```python
from build123d import *

# Parameters (mm, degrees)
SKETCH_1_W           = 100
SKETCH_1_H           = 30
SKETCH_1_R           = 1.45
EXTRUDE_1_DEPTH      = 10
SKETCH_2_W           = 24
SKETCH_2_H           = 30
CUT_EXTRUDE_1_DEPTH  = 6.5
SKETCH_3_W           = 9
SKETCH_3_H           = 15
CUT_EXTRUDE_2_DEPTH  = 16.5
SKETCH_4_W           = 9
SKETCH_4_H           = 4
CUT_EXTRUDE_3_DEPTH  = 16.5
SKETCH_6_R           = 1.5
CUT_EXTRUDE_4_DEPTH  = 16
CUT_EXTRUDE_START    = -8
SKETCH_7_R           = 1.5
CUT_EXTRUDE_5_DEPTH  = 8
CHAMFER_1_SIZE       = 5
CUT_EXTRUDE_START_2  = -30
SKETCH_10_R          = 1.5
CUT_EXTRUDE_8_DEPTH  = 30
SKETCH_11_R          = 1.5
CUT_EXTRUDE_9_DEPTH  = 30
SKETCH_15_W          = 27.5
SKETCH_15_H          = 2.5
CUT_EXTRUDE_14_DEPTH = 30
CUT_EXTRUDE_15_REACH = 106.881
SKETCH_16_W          = 9
SKETCH_16_H          = 2
SKETCH_19_R          = 1.45
CUT_EXTRUDE_18_DEPTH = 105.880884817
SKETCH_21_W          = 30
SKETCH_21_H          = 6.5
EXTRUDE_2_DEPTH      = 3
CUT_EXTRUDE_START_3  = -2
SKETCH_22_R          = 1.5
CUT_EXTRUDE_19_DEPTH = 2
SKETCH_23_W          = 30
SKETCH_23_H          = 6.5
EXTRUDE_3_DEPTH      = 3
SKETCH_24_R          = 1.5
CUT_EXTRUDE_20_DEPTH = 2


with BuildPart() as part:
    # 草图1 → 凸台-拉伸1 (new body)
    with BuildSketch(Plane(origin=(0, 0, 0), x_dir=(1, 0, 0), z_dir=(0, 1, 0))):
        with Locations((-50, 15)):
            Rectangle(SKETCH_1_W, SKETCH_1_H)
        with Locations(Location((-50, 25, 0), (0, 0, 270))):
            Circle(SKETCH_1_R, mode=Mode.SUBTRACT)
        with Locations(Location((-50, 5, 0), (0, 0, 270))):
            Circle(SKETCH_1_R, mode=Mode.SUBTRACT)
    extrude(amount=EXTRUDE_1_DEPTH)

    # 草图2 → 切除-拉伸1 (cut)
    with BuildSketch(Plane(origin=(0, 10, 0), x_dir=(1, 0, 0), z_dir=(0, 1, 0))):
        with Locations((-50, 15)):
            Rectangle(SKETCH_2_W, SKETCH_2_H)
    extrude(amount=-CUT_EXTRUDE_1_DEPTH, mode=Mode.SUBTRACT)

    # 草图3 → 切除-拉伸2 (cut)
    with BuildSketch(Plane(origin=(0, 10, 0), x_dir=(1, 0, 0), z_dir=(0, 1, 0))):
        with Locations((-68, 22.5)):
            Rectangle(SKETCH_3_W, SKETCH_3_H)
        with Locations((-32, 22.5)):
            Rectangle(SKETCH_3_W, SKETCH_3_H)
    extrude(amount=-CUT_EXTRUDE_2_DEPTH, mode=Mode.SUBTRACT)

    # 草图4 → 切除-拉伸3 (cut)
    with BuildSketch(Plane(origin=(0, 0, -15), x_dir=(-1, 0, 0), z_dir=(0, 0, -1))):
        with Locations((68, 8)):
            Rectangle(SKETCH_4_W, SKETCH_4_H)
        with Locations((32, 8)):
            Rectangle(SKETCH_4_W, SKETCH_4_H)
    extrude(amount=-CUT_EXTRUDE_3_DEPTH, mode=Mode.SUBTRACT)

    # 草图6 → 切除-拉伸4 (cut)
    with BuildSketch(Plane(origin=(-62, 0, 0), x_dir=(0, 0, -1), z_dir=(1, 0, 0))):
        with Locations((22.5, 5)):
            Circle(SKETCH_6_R)
    extrude(amount=-CUT_EXTRUDE_4_DEPTH, mode=Mode.SUBTRACT)

    # 草图7 → 切除-拉伸5 (cut)
    with BuildSketch(Plane.ZY.offset(38).offset(CUT_EXTRUDE_START)):
        with Locations(Location((-22.5, 5, 0), (0, 0, 180))):
            Circle(SKETCH_7_R)
    extrude(amount=CUT_EXTRUDE_5_DEPTH, mode=Mode.SUBTRACT)

    # 倒角1
    chamfer_1_edges = [part.edges().sort_by_distance(p)[0] for p in [
        (-32, 6, -15),
        (-68, 6, -15),
    ]]
    chamfer(chamfer_1_edges, length=CHAMFER_1_SIZE)

    # 草图10 → 切除-拉伸8 (cut)
    with BuildSketch(Plane(origin=(-100, -149.284504662, 244.723777946), x_dir=(0, 0, 1), z_dir=(-1, 0, 0)).offset(CUT_EXTRUDE_START_2)):
        with Locations(Location((-267.223777946, 154.284504662, 0), (0, 0, 180))):
            Circle(SKETCH_10_R)
    extrude(amount=CUT_EXTRUDE_8_DEPTH, mode=Mode.SUBTRACT)

    # 草图11 → 切除-拉伸9 (cut)
    with BuildSketch(Plane(origin=(0, -149.284504662, 244.723777946), x_dir=(0, 0, -1), z_dir=(1, 0, 0))):
        with Locations((267.223777946, 154.284504662)):
            Circle(SKETCH_11_R)
    extrude(amount=-CUT_EXTRUDE_9_DEPTH, mode=Mode.SUBTRACT)

    # 草图15 → 切除-拉伸14 (cut)
    with BuildSketch(Plane(origin=(0, 0, -30), x_dir=(-1, 0, 0), z_dir=(0, 0, -1))):
        with Locations((13.75, 8.75)):
            Rectangle(SKETCH_15_W, SKETCH_15_H)
        with Locations((86.25, 8.75)):
            Rectangle(SKETCH_15_W, SKETCH_15_H)
    extrude(amount=-CUT_EXTRUDE_14_DEPTH, mode=Mode.SUBTRACT)

    # 切除-拉伸15: up to this plane
    cut_extrude_15_end = Plane(origin=(-63.5, 6, -10), z_dir=(0, -0.7071067811865456, 0.7071067811865495))
    # 草图16 → 切除-拉伸15 (cut, up to the surface)
    with BuildSketch(Plane.XY, mode=Mode.PRIVATE) as cut_extrude_15_sk1:
        with Locations((-68, 1)):
            Rectangle(SKETCH_16_W, SKETCH_16_H)
    cut_extrude_15_tool1 = split(extrude(cut_extrude_15_sk1.sketch, amount=-CUT_EXTRUDE_15_REACH, mode=Mode.PRIVATE), bisect_by=cut_extrude_15_end, keep=Keep.BOTH, mode=Mode.PRIVATE)
    add(cut_extrude_15_tool1.solids().sort_by_distance((-68, 1, 0))[0], mode=Mode.SUBTRACT)
    # 草图16 → 切除-拉伸15 (cut, up to the surface)
    with BuildSketch(Plane.XY, mode=Mode.PRIVATE) as cut_extrude_15_sk2:
        with Locations((-32, 1)):
            Rectangle(SKETCH_16_W, SKETCH_16_H)
    cut_extrude_15_tool2 = split(extrude(cut_extrude_15_sk2.sketch, amount=-CUT_EXTRUDE_15_REACH, mode=Mode.PRIVATE), bisect_by=cut_extrude_15_end, keep=Keep.BOTH, mode=Mode.PRIVATE)
    add(cut_extrude_15_tool2.solids().sort_by_distance((-32, 1, 0))[0], mode=Mode.SUBTRACT)

    # 草图19 → 切除-拉伸18 (cut, through all)
    with BuildSketch(Plane.XZ):
        with Locations(Location((-3, -3, 0), (0, 0, 270))):
            Circle(SKETCH_19_R)
        with Locations(Location((-17, -3, 0), (0, 0, 270))):
            Circle(SKETCH_19_R)
        with Locations(Location((-17, -27, 0), (0, 0, 270))):
            Circle(SKETCH_19_R)
        with Locations(Location((-3, -27, 0), (0, 0, 270))):
            Circle(SKETCH_19_R)
        with Locations((-97, -27)):
            Circle(SKETCH_19_R)
        with Locations((-83, -27)):
            Circle(SKETCH_19_R)
        with Locations((-83, -3)):
            Circle(SKETCH_19_R)
        with Locations((-97, -3)):
            Circle(SKETCH_19_R)
    extrude(amount=-CUT_EXTRUDE_18_DEPTH, mode=Mode.SUBTRACT)

    # 草图21 → 凸台-拉伸2 (add)
    with BuildSketch(Plane(origin=(-62, 0, 0), x_dir=(0, 0, -1), z_dir=(1, 0, 0))):
        with Locations((15, 6.75)):
            Rectangle(SKETCH_21_W, SKETCH_21_H)
    extrude(amount=EXTRUDE_2_DEPTH)

    # 草图22 → 切除-拉伸19 (cut)
    with BuildSketch(Plane.ZY.offset(62).offset(CUT_EXTRUDE_START_3)):
        with Locations(Location((-22.5, 5, 0), (0, 0, 180))):
            Circle(SKETCH_22_R)
    extrude(amount=CUT_EXTRUDE_19_DEPTH, mode=Mode.SUBTRACT)

    # 草图23 → 凸台-拉伸3 (add)
    with BuildSketch(Plane.ZY.offset(38)):
        with Locations((-15, 6.75)):
            Rectangle(SKETCH_23_W, SKETCH_23_H)
    extrude(amount=EXTRUDE_3_DEPTH)

    # 草图24 → 切除-拉伸20 (cut)
    with BuildSketch(Plane(origin=(-38, 0, 0), x_dir=(0, 0, -1), z_dir=(1, 0, 0))):
        with Locations((22.5, 5)):
            Circle(SKETCH_24_R)
    extrude(amount=-CUT_EXTRUDE_20_DEPTH, mode=Mode.SUBTRACT)


solid = part.part
```
Model file for the job. Use its own axes, mm. A direction names the side the tool comes from. Coordinates: 2 decimals unless noted, no trailing zeros. Write each loop counter-clockwise with the first axis right and the second up, starting at its lowest first coordinate (ties: lowest second). Pieces come first, ordered by that corner, then holes. Notation, with made-up numbers: (-28, 46) - (31, 46) arc R27 ccw to (31, 85) - close; hole circle Ø4 at (45, 38.25). An arc over 180 degrees is marked (long way). One line per item, written item: value. Start each with the question number.
1. Slice it at A-A (z = -16.75). Write the cut outline in (x, y).
2. Slice it at C-C (x = -3). Write the cut outline in (y, z).
3. Mould opens along X. For faces 5 (the flat face through (0, 4, -15)), 6 (the flat face through (-72.5, 4, -18)), 7 (the flat face through (-50, 3, -30)) say: released by +X, released by -X, zero draft, split by the parting line, or undercut.
4. Flat gauge pins, fed straight in: pin 1 (2.5 mm diameter, centred on y = 5, z = -22.5, fed in from +X); pin 2 (4.5 mm diameter, centred on x = -66.5, z = -5, fed in from +Y); pin 3 (6 mm diameter, centred on x = -44.5, z = -25.5, fed in from +Y); pin 4 (2.5 mm diameter, centred on x = -97, z = -3, fed in from -Y). Where does each tip first touch, or does it go through?
5. Tool access for faces 1 (the flat face through (-60, 5, -22)), 2 (the cylindrical face through (-14, 5, -21)), 3 (the flat face through (-32, 4, -12)), 4 (the flat face through (-50, 3.5, -15)): list every direction of +Z, -Z, +X, -X, +Y, -Y with a clear straight run to the whole face (end or side of a thin tool).
6. Slice it at D-D (z = -22.25). Count the separate pieces of the cut face and the enclosed holes in it, plus the area to 3 significant figures.
7. Slice it at B-B (x = -50). Write the cut outline in (y, z), plus the area to 3 significant figures.
8. Probe line 1 (X direction, y = 5, z = -16); line 2 (X direction, y = 1.25, z = -17.25); line 3 (X direction, y = 9.25, z = -6.25). List the from-to ranges inside material, lowest first. Write a range as from..to.
Answers below:
1. outline: (-100, 0) - (-72.5, 0) - (-72.5, 7.5) - (-100, 7.5) - close; (-63.5, 0) - (-36.5, 0) - (-36.5, 10) - (-41, 10) - (-41, 3.5) - (-59, 3.5) - (-59, 10) - (-63.5, 10) - close; (-27.5, 0) - (0, 0) - (0, 7.5) - (-27.5, 7.5) - close
2. outline: (0, -30) - (7.5, -30) - (7.5, -28.45) - (0, -28.45) - close; (0, -25.55) - (7.5, -25.55) - (7.5, -4.45) - (0, -4.45) - close; (0, -1.55) - (7.5, -1.55) - (7.5, 0) - (0, 0) - close; hole circle Ø3 at (5, -22.5)
3. face 5: released by +X
3. face 6: undercut
3. face 7: zero draft
4. pin 1: stops at x = -40
4. pin 2: stops at y = 6
4. pin 3: stops at y = 3.5
4. pin 4: passes through
5. face 1: -X
5. face 2: +X
5. face 3: -Z, +Y
5. face 4: +Z, -Z, +Y
6. separate pieces: 5
6. enclosed holes: 0
6. area: 382 mm^2
7. outline: (0, -30) - (3.5, -30) - (3.5, -26.45) - (0, -26.45) - close; (0, -23.55) - (3.5, -23.55) - (3.5, -6.45) - (0, -6.45) - close; (0, -3.55) - (3.5, -3.55) - (3.5, 0) - (0, 0) - close
7. area: 84.7 mm^2
8. line 1: x = -100..-72.5, -63.5..-59, -41..-36.5, -27.5..0
8. line 2: x = -100..-72.5, -63.5..-36.5, -27.5..0
8. line 3: x = -63.5..-59, -41..-36.5
